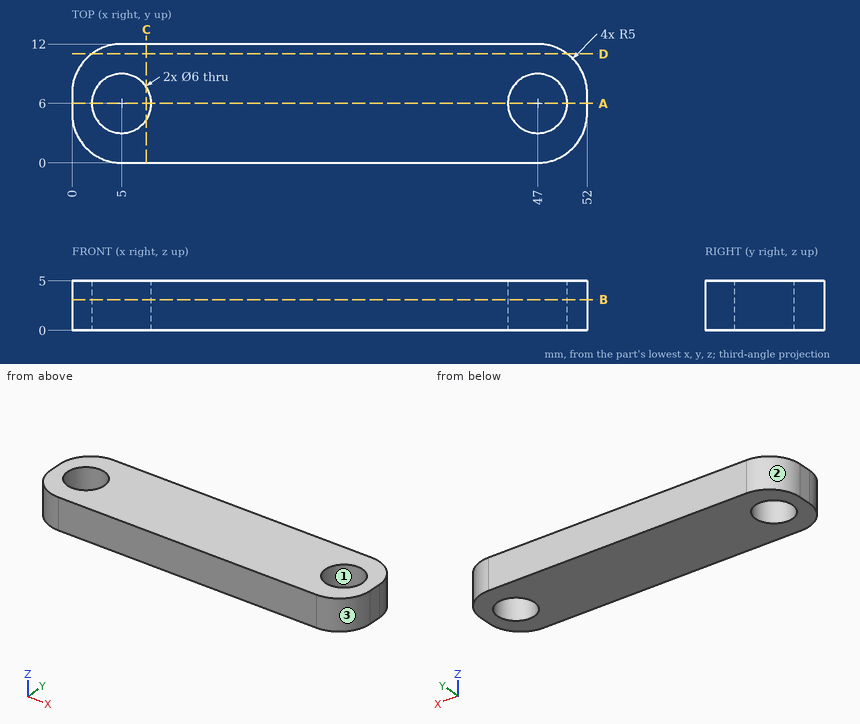
Verification items for this drawing (mm, ordinates from the low corner). Coordinates: 2 decimals unless noted, no trailing zeros. Loops run counter-clockwise (first coordinate to the right, second up) from the corner with the lowest first, then second, coordinate; pieces in that order, holes last. Notation, with made-up numbers: (58, -40) - (83, -40) arc R9 cw to (83, -28) - close; hole circle Ø3 at (0.25, 48). An arc over 180 degrees is marked (long way). Answer as a JSON object with one key per item and string values.
(1) Go/stop test with flat-tipped pins: pin 1 Ø5 at (x, y) = (47, 6) entering from -Z; pin 2 Ø1 at (y, z) = (3.5, 3) entering from +X. Record where each tip stops, or that it passes through.
Response:
{"pin 1": "passes through", "pin 2": "stops at x = 51.9"}
(2) Cross-section at D-D, the plane y = 11. Record the boundary of the cut face in (x, z).
Response:
{"outline": "(2, 0) - (50, 0) - (50, 5) - (2, 5) - close"}
(3) Scan lines: line 1 along Y through (x, z) = (5, 2.35); line 2 along X through (y, z) = (7.5, 3.2); line 3 along X through (y, z) = (5.25, 4.3). Record each from-to range of solid material in increasing order.
Response:
{"line 1": "y = 0 to 3, 9 to 12", "line 2": "x = 0.03 to 2.4, 7.6 to 44.4, 49.6 to 51.97", "line 3": "x = 0 to 2.1, 7.9 to 44.1, 49.9 to 52"}
(4) Mould release check, pull along Y, two halves, no side actions. Record for the marked faces 1, 2 and 3: pulls with the +Y half, pulls with the -Y half, needs draft (parallel to the pull), parting line crosses it, or undercut.
Response:
{"face 1": "undercut", "face 2": "pulls with the +Y half", "face 3": "pulls with the -Y half"}
(5) Cross-section at B-B, the plane z = 3.1. Record the boundary of the cut face in (x, y).
Response:
{"outline": "(0, 5) arc R5 ccw to (5, 0) - (47, 0) arc R5 ccw to (52, 5) - (52, 7) arc R5 ccw to (47, 12) - (5, 12) arc R5 ccw to (0, 7) - close; hole circle Ø6 at (5, 6); hole circle Ø6 at (47, 6)"}
(6) Cross-section at C-C, the plane x = 7.5. Record the boundary of the cut face in (y, z), then the cut area to 3 significant figures.
Response:
{"outline": "(0, 0) - (4.34, 0) - (4.34, 5) - (0, 5) - close; (7.66, 0) - (12, 0) - (12, 5) - (7.66, 5) - close", "area": "43.4 mm²"}
(7) Cross-section at A-A, the plane y = 6. Record the boundary of the cut face in (x, z), then the cut area to 3 significant figures.
Response:
{"outline": "(0, 0) - (2, 0) - (2, 5) - (0, 5) - close; (8, 0) - (44, 0) - (44, 5) - (8, 5) - close; (50, 0) - (52, 0) - (52, 5) - (50, 5) - close", "area": "200 mm²"}
